Autodesk Inventor part; units mm, degrees
ref_plane "YZ Plane" through (0, 0, 0) normal (1, 0, 0) x (0, 1, 0)
ref_plane "XZ Plane" through (0, 0, 0) normal (0, 1, 0) x (-1, 0, 0)
ref_plane "XY Plane" through (0, 0, 0) normal (0, 0, 1) x (1, 0, 0)
sketch "草圖1" plane through (0, 0, 0) normal (0, 1, 0) x (-1, 0, 0)
  line L0 (-25, 27) -> (-25, -27)
  line L1 (-25, -30) -> (24.1827, -30)
  line L2 (17.3, 27) -> (11.3, 27)
  line L3 (11.3, 27) -> (11.3, 24)
  line L4 (11.3, 24) -> (17.3, 24)
  line L5 (17.3, 24) -> (17.3, 27)
  line L6 (17.3, 22.5) -> (14.3, 22.5)
  line L7 (14.3, 22.5) -> (14.3, 12.5)
  line L8 (14.3, 12.5) -> (17.3, 12.5)
  line L9 (17.3, 12.5) -> (17.3, 22.5)
  line L10 (14.3, 12.5) -> (15.8, 12.5)
  circle A0 centre (15.8, 0) radius 1.5
  line L11 (14.3, -22.5) -> (17.3, -22.5)
  line L12 (17.3, -22.5) -> (17.3, -12.5)
  line L13 (17.3, -12.5) -> (14.3, -12.5)
  line L14 (14.3, -12.5) -> (14.3, -22.5)
  circle A1 centre (7.8, 25.5) radius 1.5
  line L15 (-1.7, 24) -> (4.3, 24)
  line L16 (4.3, 24) -> (4.3, 27)
  line L17 (4.3, 27) -> (-1.7, 27)
  line L18 (-1.7, 27) -> (-1.7, 24)
  line L19 (-6.7, 21) -> (-18.7, 21)
  line L20 (-18.7, 21) -> (-18.7, -2)
  line L21 (-18.7, -2) -> (-6.7, -2)
  line L22 (-6.7, -2) -> (-6.7, 21)
  line L23 (-6.7, 21) -> (-6.7, 9.5)
  circle A2 centre (-3.7, 9.5) radius 1.5
  circle A3 centre (-21.7, 9.5) radius 1.5
  line L24 (-2.5, -19.8) -> (-12.5, -19.8)
  line L25 (-12.5, -19.8) -> (-12.5, -22.8)
  line L26 (-12.5, -22.8) -> (-2.5, -22.8)
  line L27 (-2.5, -22.8) -> (-2.5, -19.8)
  line L28 (-25, -30) -> (-25, -27)
  line L29 (-12.5, -22.8) -> (-12.5, -21.3)
  line L30 (25, 30) -> (25, -30)
  line L31 (25, -30) -> (24.1827, -30)
  line L32 (25, 30) -> (25, 27)
  line L33 (-25, 30) -> (-25, 27)
  line L34 (0, -42) -> (0, 42)
  line L35 (35, 0) -> (-35, 0)
  line L36 (25, 30) -> (25, 27)
  line L37 (25, 30) -> (-25, 30)
  point P0 (25, -30)
  dimension "d1" = 50
  dimension "d46" = 3
  dimension "d47" = 1.5
  dimension "d48" = 3
  dimension "d49" = 10
  dimension "d50" = 3
  dimension "d51" = 1.5
  dimension "d53" = 3
  dimension "d54" = 3
  dimension "d55" = 10
  dimension "d56" = 3
  dimension "d61" = 3
  dimension "d62" = 6
  dimension "d63" = 3
  dimension "d67" = 12
  dimension "d68" = 23
  dimension "d69" = 11.5
  dimension "d72" = 3
  dimension "d73" = 3
  dimension "d74" = 10
  dimension "d75" = 3
  dimension "d88" = 60
  dimension "d91" = 25
  dimension "d92" = 30
extrude "擠出2" add sketch "草圖1" along normal mid plane 3 contours L33 L37 L34 L17 L18 L15 L35 L22 L19 L20 L0 | L35 L20 L21 L22 L34 L1 L28 L0 | L37 L30 L35 A0 L34 L15 L16 L17 | L34 L35 A0 L30 L31 L1
fillet "圓角1" radius 3 4 edges at (-25, 0, 30) (25, 0, 30) (-25, 0, -30) (25, 0, -30)
properties part number "板子1"
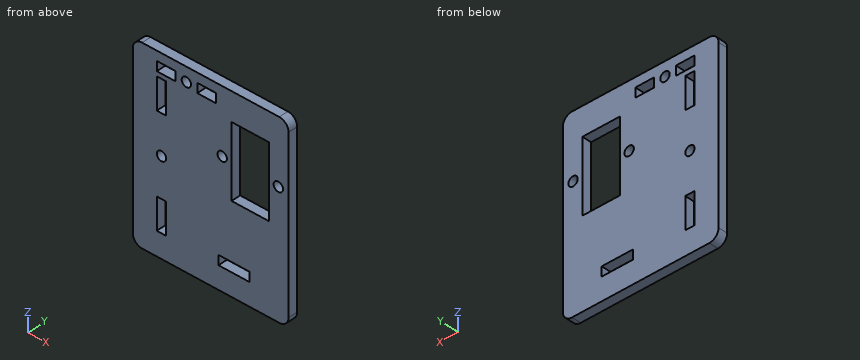
The listing builds one solid part. Answer for the finished solid, in the listing's coordinates (mm). Round coordinates to 2 decimals unless told otherwise and drop trailing zeros. Loops run counter-clockwise (first coordinate to the right, second up) from the corner with the lowest first, then second, coordinate; pieces in that order, holes last.
1) A cutting plane is placed at C-C on z = 25.5. Determine the outline of the cut face in (x, y).
Outcome:
outline: (-25, -1.5) - (-17.3, -1.5) - (-17.3, 1.5) - (-25, 1.5) - close; (-11.3, -1.5) - (-9.3, -1.5) - (-9.3, 1.5) - (-11.3, 1.5) - close; (-6.3, -1.5) - (-4.3, -1.5) - (-4.3, 1.5) - (-6.3, 1.5) - close; (1.7, -1.5) - (25, -1.5) - (25, 1.5) - (1.7, 1.5) - close
2) A cutting plane is placed at D-D on z = 0. Determine the outline of the cut face in (x, y), plus the area to 3 significant figures.
Outcome:
outline: (-25, -1.5) - (-17.3, -1.5) - (-17.3, 1.5) - (-25, 1.5) - close; (-14.3, -1.5) - (6.7, -1.5) - (6.7, 1.5) - (-14.3, 1.5) - close; (18.7, -1.5) - (25, -1.5) - (25, 1.5) - (18.7, 1.5) - close
area: 105 mm2
3) Consider line 1 (X direction, y = 0.9, z = -22); line 2 (X direction, y = -0.4, z = 13); line 3 (Z direction, x = -15.8, y = -0.65). Determine where each line is inside the solid, lowest interval first.
Outcome:
line 1: x = -25 to -17.3, -14.3 to 2.5, 12.5 to 25
line 2: x = -25 to -17.3, -14.3 to 6.7, 18.7 to 25
line 3: z = -30 to -22.5, -12.5 to -1.5, 1.5 to 12.5, 22.5 to 24, 27 to 30
4) A cutting plane is placed at B-B on x = 3.7. Determine the outline of the cut face in (y, z).
Outcome:
outline: (-1.5, -30) - (1.5, -30) - (1.5, -22.8) - (-1.5, -22.8) - close; (-1.5, -19.8) - (1.5, -19.8) - (1.5, 8) - (-1.5, 8) - close; (-1.5, 11) - (1.5, 11) - (1.5, 30) - (-1.5, 30) - close
5) A cutting plane is placed at A-A on x = -15.8. Determine the outline of the cut face in (y, z), plus the area to 3 significant figures.
Outcome:
outline: (-1.5, -30) - (1.5, -30) - (1.5, -22.5) - (-1.5, -22.5) - close; (-1.5, -12.5) - (1.5, -12.5) - (1.5, -1.5) - (-1.5, -1.5) - close; (-1.5, 1.5) - (1.5, 1.5) - (1.5, 12.5) - (-1.5, 12.5) - close; (-1.5, 22.5) - (1.5, 22.5) - (1.5, 24) - (-1.5, 24) - close; (-1.5, 27) - (1.5, 27) - (1.5, 30) - (-1.5, 30) - close
area: 102 mm2
